Geometry check sheet. Reference: the model listing, model coordinates, mm. A direction names the side the tool comes from. Give positions to 0.01 mm unless a question says otherwise; leave off trailing zeros. Write each loop counter-clockwise with the first axis right and the second up, starting at its lowest first coordinate (ties: lowest second). Pieces come first, ordered by that corner, then holes. Notation, with made-up numbers: (70, -21.75) - (84, -21.75) arc R20 ccw to (84, -12.75) - close; hole circle Ø10 at (63, 37.5). An arc over 180 degrees is marked (long way). Use a Markdown table: item, result.
```python
from build123d import *

# Parameters (mm, degrees)
F0_R     = 3.75
F0_R_2   = 1.75
F1_DEPTH = 10
F0_W     = 30
F0_H     = 30
F2_DEPTH = 2
F3_DEPTH = 10


with BuildPart() as f1:
    # F0 (on Top) → F1 (new body)
    with BuildSketch(Plane.XY):
        Circle(F0_R)
        Circle(F0_R_2, mode=Mode.SUBTRACT)
    extrude(amount=F1_DEPTH)

    # F0 (on Top) → F2 (join)
    with BuildSketch(Plane.XY):
        Rectangle(F0_W, F0_H)
        Circle(F0_R, mode=Mode.SUBTRACT)
        Polygon((17, 15), (15, 15), (15, -15), (-15, -15), (-15, -17), (17, -17), align=None)
    extrude(amount=F2_DEPTH)

    # F0 (on Top) → F3 (join)
    with BuildSketch(Plane.XY):
        Polygon((17, 15), (15, 15), (15, -15), (-15, -15), (-15, -17), (17, -17), align=None)
    extrude(amount=-F3_DEPTH)


solid = f1.part
```
1) Section check A-A on x = 0. Record the boundary of the cut face in (y, z).
Working result:
| item | result |
|---|---|
| outline | (-17, -10) - (-15, -10) - (-15, 0) - (-1.75, 0) - (-1.75, 10) - (-3.75, 10) - (-3.75, 2) - (-17, 2) - close; (1.75, 0) - (15, 0) - (15, 2) - (3.75, 2) - (3.75, 10) - (1.75, 10) - close |
2) Set-up check for faces 1 (the flat face through (-15, -4.5, 0.4)), 2 (the flat face through (-4, 0, 0)): record each of +Z, -Z, +X, -X, +Y, -Y from which the full face is reachable in a straight line by a thin tool's end or side.
Working result:
| item | result |
|---|---|
| face 1 | +Z, -Z, -X, +Y, -Y |
| face 2 | -Z, -X, +Y |
3) Mould release check, pull along X, two halves, no side actions. Record for faces 3 (the cylindrical face through (1.617, -0.67, 4.93)), 4 (the flat face through (17, -1, -4)), 5 (the cylindrical face through (-3.746, 0.165, 5.944)), 6 (the flat face through (0, -15, -5)): pulls with the +X half, pulls with the -X half, needs draft (parallel to the pull), parting line crosses it, or undercut.
Working result:
| item | result |
|---|---|
| face 3 | undercut |
| face 4 | pulls with the +X half |
| face 5 | parting line crosses it |
| face 6 | needs draft |
4) Depth check by flat-ended pin: P1, Ø10, axis at x = 13, y = -13.5, coming from the +Z side; P2, Ø12, axis at y = -10, z = -2.5, coming from the -X side; P3, Ø2, axis at x = 3, z = 5.5, coming from the +Y side; P4, Ø2, axis at x = 10, y = -0.5, coming from the -Z side. Enter the tip coordinate at first touch or a pass-through.
Working result:
| item | result |
|---|---|
| P1 | stops at z = 2 |
| P2 | stops at x = -15 |
| P3 | stops at y = 3.17 |
| P4 | stops at z = 0 |
5) Material ranges on L1, parallel to Y at x = 0, z = 7; L2, parallel to Y at x = -11.5, z = -0.75; L3, parallel to Z at x = 14.5, y = -9, recorded low to high. Write a range as from..to.
Working result:
| item | result |
|---|---|
| L1 | y = -3.75..-1.75, 1.75..3.75 |
| L2 | y = -17..-15 |
| L3 | z = 0..2 |
6) Section check B-B on y = 0. Record the boundary of the cut face in (x, z), then the cut area to 3 significant figures.
Working result:
| item | result |
|---|---|
| outline | (-15, 0) - (-1.75, 0) - (-1.75, 10) - (-3.75, 10) - (-3.75, 2) - (-15, 2) - close; (1.75, 0) - (15, 0) - (15, -10) - (17, -10) - (17, 2) - (3.75, 2) - (3.75, 10) - (1.75, 10) - close |
| area | 109 mm² |
7) Section check D-D on z = -4. Record the boundary of the cut face in (x, y).
Working result:
| item | result |
|---|---|
| outline | (-15, -17) - (17, -17) - (17, 15) - (15, 15) - (15, -15) - (-15, -15) - close |
8) Section check C-C on y = 5. Record the boundary of the cut face in (x, z), then the cut area to 3 significant figures.
Working result:
| item | result |
|---|---|
| outline | (-15, 0) - (15, 0) - (15, -10) - (17, -10) - (17, 2) - (-15, 2) - close |
| area | 84.0 mm² |
